Source: CAD feature listing. Evaluate the final solid. Frame: model axes, mm. A direction names the side the tool comes from. Round coordinates to 2 decimals unless told otherwise and drop trailing zeros. Order: outer loops, then holes, each group sorted by start corner. A loop starts at its lowest first (then second) coordinate and runs counter-clockwise, first axis right, second up. Notation, with made-up numbers: M 39,64 L 67,64 A20 cw 67,103 Z; hole C 72,61.5 d3. An arc over 180 degrees is marked long. Answer as CSV lines item,"result". Start each with the question number.
Item 1: Line query: line 1 (Z direction, x = -1.15, y = -1.45); line 2 (Y direction, x = 0.45, z = -2); line 3 (X direction, y = -0.65, z = 2). Output: solid intervals per line, ascending. Write a range as [from, to].
Item 2: Section query B-B on z = -3. Return the cut outline in (x, y).
Item 3: Set-up query: faces 1 (the face through (0, 0, -6)), 2 (the face through (0.87, -0.49, 1.96)), 3 (the face through (0.5, -1.5, 0)). Return all of +Z, -Z, +X, -X, +Y, -Y with unobstructed straight access to the full face (end or side cutting, diameter ignored); none if empty.
Solid Edge part; units mm, degrees
sketch "Sketch1" plane through (0, 0, 0) normal (0, 0, 1) x (1, 0, 0)
  circle A0 centre (0, 0) radius 2.25
extrude "Protrusion1" add sketch "Sketch1" along normal blind 2.5
sketch "Sketch2" plane through (0, 0, 2.5) normal (0, 0, 1) x (0, 1, 0)
  line L0 (0, 1.1547) -> (1, 0.5774)
  line L1 (1, 0.5774) -> (1, -0.5774)
  line L2 (1, -0.5774) -> (0, -1.1547)
  line L3 (0, -1.1547) -> (-1, -0.5774)
  line L4 (-1, -0.5774) -> (-1, 0.5774)
  line L5 (-1, 0.5774) -> (0, 1.1547)
extrude "Cutout1" cut sketch "Sketch2" against normal blind 1.1
fillet "Round1" radius 0.25 1 edges at (-2.25, 0, 2.5)
sketch "Sketch3" plane through (0, 0, 0) normal (1, 0, 0) x (0, 1, 0)
  line L0 (-0.974, -6) -> (0, -6)
  line L1 (-1.25, -5.724) -> (-0.974, -6)
  line L2 (-1.25, -1.35) -> (-1.25, -5.724)
  line L3 (-0.974, -1.35) -> (-1.25, -1.35)
  line L4 (-0.974, -1.34) -> (-0.974, -1.35)
  line L5 (-1.25, -1.34) -> (-0.974, -1.34)
  line L6 (-1.25, -0.1) -> (-1.25, -1.34)
  arc A0 (-1.25, -0.1) -> (-1.35, 0) centre (-1.35, -0.1) ccw
revolve "RevolvedProtrusion1" add sketch "Sketch3" angle 360 about axis through (0, 0, -60.325) along (0, 0, 1) material side at (0, -0.487, -5.95)
cosmetic_thread "Thread1"
sketch "Sketch4" plane through (0, 0, 0) normal (0, -1, 0) x (1, 0, 0)
  line L0 (-1.15, 2.5) -> (0, 1.836)
revolve "RevolvedCutout1" cut sketch "Sketch4" angle 360 about axis through (0, 0, 57.15) along (0, 0, -1) material side at (-0.55, 0, 2.2113)
properties material "Stahl"
Results:
1,line 1,"[0, 2.5]"
1,line 2,"[-1.17, 1.17]"
1,line 3,"[-2.15, -0.78], [0.78, 2.15]"
2,outline,"C 0,0 d2.5"
3,face 1,"-Z, +X, -X, +Y, -Y"
3,face 2,"+Z"
3,face 3,"-Z"
